from build123d import *

# Parameters (mm, degrees)
SKETCH1_W      = 165.1
SKETCH1_H      = 165.1
SKETCH1_R      = 6.35
SKETCH1_R_2    = 4.7625
EXTRUDE1_DEPTH = 3.175


with BuildPart() as part:
    # Sketch1 → Extrude1 (new body)
    with BuildSketch(Plane(origin=(0, 0, 0), x_dir=(1, 0, 0), z_dir=(0, 1, 0))):
        Rectangle(SKETCH1_W, SKETCH1_H)
        Circle(SKETCH1_R, mode=Mode.SUBTRACT)
        with Locations((-69.40042, 69.40042)):
            Circle(SKETCH1_R_2, mode=Mode.SUBTRACT)
        with Locations((69.40042, 69.40042)):
            Circle(SKETCH1_R_2, mode=Mode.SUBTRACT)
        with Locations((69.40042, -69.40042)):
            Circle(SKETCH1_R_2, mode=Mode.SUBTRACT)
        with Locations((-69.40042, -69.40042)):
            Circle(SKETCH1_R_2, mode=Mode.SUBTRACT)
    extrude(amount=-EXTRUDE1_DEPTH)


solid = part.part
Can you work these out from the model? Positions are in its coordinate system, mm. Round coordinates to 2 decimals unless told otherwise and drop trailing zeros. Loops run counter-clockwise (first coordinate to the right, second up) from the corner with the lowest first, then second, coordinate; pieces in that order, holes last. Notation, with made-up numbers: (55, 77) - (70, 77) arc R17 cw to (70, 90) - close; hole circle Ø4 at (82.25, -11.5). An arc over 180 degrees is marked (long way). Use CSV: the item, a comma, the result in double quotes. Start each with the question number.
1) For pin 1 Ø7.5 at (x, z) = (-69.4, 69.4) entering from +Y, with a flat end and sliding along its axis, tell me the tip position at first contact or that it passes through.
2) We'd pull the mould along X, two halves only. Please class faces 1 (the cylindrical face through (68.78, -1.565, -74.122)), 2 (the flat face through (-1, 0, -20)): released by +X, released by -X, zero draft, split by the parting line, or undercut.
3) If we section it at B-B on z = 0: Write out the boundary of the cut face in (x, y) (3 decimals).
4) If we section it at A-A on x = 0: Write out the boundary of the cut face in (y, z) (3 decimals), plus the area to 3 significant figures.
5) Please list where these lines run through material, in increasing order: probe 1 along Z at (x, y) = (-69.5, -0.25); probe 2 along X at (y, z) = (-1.35, 0); probe 3 along Z at (x, y) = (68, -0.7). Write a range as [from, to].
6) If we section it at D-D on z = 67: Write out the boundary of the cut face in (x, y) (3 decimals).
7) If we section it at C-C on y = -2.45: Count the separate pieces of the cut face and the enclosed holes in it, plus the area to 3 significant figures.
Geometry results:
1,pin 1,"passes through"
2,face 1,"undercut"
2,face 2,"zero draft"
3,outline,"(-82.55, -3.175) - (-6.35, -3.175) - (-6.35, 0) - (-82.55, 0) - close; (6.35, -3.175) - (82.55, -3.175) - (82.55, 0) - (6.35, 0) - close"
4,outline,"(-3.175, -82.55) - (0, -82.55) - (0, -6.35) - (-3.175, -6.35) - close; (-3.175, 6.35) - (0, 6.35) - (0, 82.55) - (-3.175, 82.55) - close"
4,area,"484 mm2"
5,probe 1,"z = [-82.55, -74.16], [-64.64, 64.64], [74.16, 82.55]"
5,probe 2,"x = [-82.55, -6.35], [6.35, 82.55]"
5,probe 3,"z = [-82.55, -73.95], [-64.85, 64.85], [73.95, 82.55]"
6,outline,"(-82.55, -3.175) - (-73.514, -3.175) - (-73.514, 0) - (-82.55, 0) - close; (-65.287, -3.175) - (65.287, -3.175) - (65.287, 0) - (-65.287, 0) - close; (73.514, -3.175) - (82.55, -3.175) - (82.55, 0) - (73.514, 0) - close"
7,separate pieces,"1"
7,enclosed holes,"5"
7,area,"26,800 mm2"
